```python
from build123d import *

# Parameters (mm, degrees)
SKETCH1_W           = 79.375
SKETCH1_H           = 44.45
BOSS_EXTRUDE1_DEPTH = 3.175
SKETCH2_W           = 3.175
SKETCH2_H           = 19.05
BOSS_EXTRUDE2_DEPTH = 3.175
SKETCH5_W           = 19.05
SKETCH5_H           = 3.175
BOSS_EXTRUDE3_DEPTH = 3.175
SKETCH3_W           = 3.175
SKETCH3_H           = 19.05
CUT_EXTRUDE1_DEPTH  = 3.175
SKETCH6_W           = 0.762
SKETCH6_H           = 19.05
BOSS_EXTRUDE4_DEPTH = 3.175
SKETCH7_R           = 1.524
CUT_EXTRUDE2_DEPTH  = 93.620796126


with BuildPart() as part:
    # Sketch1 → Boss-Extrude1 (new body)
    with BuildSketch(Plane.XY):
        with Locations((39.6875, 22.225)):
            Rectangle(SKETCH1_W, SKETCH1_H)
    extrude(amount=BOSS_EXTRUDE1_DEPTH)

    # Sketch2 → Boss-Extrude2 (add)
    with BuildSketch(Plane.XY.offset(3.175)):
        with Locations((-1.5875, 22.225)):
            Rectangle(SKETCH2_W, SKETCH2_H)
    extrude(amount=-BOSS_EXTRUDE2_DEPTH)

    # Sketch5 → Boss-Extrude3 (add)
    with BuildSketch(Plane.XY.offset(3.175)):
        with Locations((38.1, 46.0375)):
            Rectangle(SKETCH5_W, SKETCH5_H)
        with Locations((38.1, -1.5875)):
            Rectangle(SKETCH5_W, SKETCH5_H)
    extrude(amount=-BOSS_EXTRUDE3_DEPTH)

    # Sketch3 → Cut-Extrude1 (cut)
    with BuildSketch(Plane.XY.offset(3.175)):
        with Locations((77.7875, 22.225)):
            Rectangle(SKETCH3_W, SKETCH3_H)
    extrude(amount=-CUT_EXTRUDE1_DEPTH, mode=Mode.SUBTRACT)

    # Sketch6 → Boss-Extrude4 (add)
    with BuildSketch(Plane.XY.offset(3.175)):
        with Locations((-3.556, 22.225)):
            Rectangle(SKETCH6_W, SKETCH6_H)
    extrude(amount=-BOSS_EXTRUDE4_DEPTH)

    # Sketch7 → Cut-Extrude2 (cut, through all)
    with BuildSketch(Plane.XY.offset(3.175)):
        with Locations((-1.5875, 22.225)):
            Circle(SKETCH7_R)
    extrude(amount=-CUT_EXTRUDE2_DEPTH, mode=Mode.SUBTRACT)


solid = part.part
```
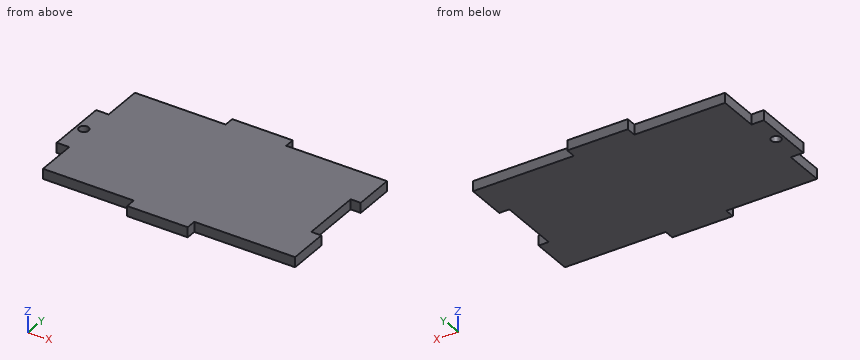
Could you check a few things on this model? Use its own coordinates, in mm. Round coordinates to 2 decimals unless told otherwise and drop trailing zeros. Loops run counter-clockwise (first coordinate to the right, second up) from the corner with the lowest first, then second, coordinate; pieces in that order, holes last.
Q1. Please list where these lines run through material, in increasing order: L1, parallel to X at y = 27, z = 1.2; L2, parallel to Y at x = 74, z = 1.5; L3, parallel to X at y = 12, z = 2.3 (3 decimals).
Q2. I want a section at C-C (y = 39.5). Write out the boundary of the cut face in (x, z) (3 decimals).
Q3. For P1, Ø1, axis at x = 17.5, z = 2.5, coming from the -Y side; P2, Ø1.6, axis at y = 25.5, z = 2.5, coming from the +X side; P3, Ø1.6, axis at x = 77.5, z = 1.5, coming from the +Y side; P4, Ø2.5, axis at x = -1.59, y = 22.22, coming from the -Z side, each with a flat end and sliding along its axis, tell me the tip position at first contact or that it passes through.
Q4. I want a section at B-B (x = 27). Write out the boundary of the cut face in (y, z) (3 decimals).
Answer below:
1. L1: x = -3.94 to 76.2
1. L2: y = 0 to 44.45
1. L3: x = 0 to 79.375
2. outline: (0, 0) - (79.375, 0) - (79.375, 3.175) - (0, 3.175) - close
3. P1: stops at y = 0
3. P2: stops at x = 76.2
3. P3: stops at y = 44.45
3. P4: passes through
4. outline: (0, 0) - (44.45, 0) - (44.45, 3.175) - (0, 3.175) - close
